Source: CAD feature listing. Evaluate the final solid. Frame: model axes, mm. Give positions to 0.01 mm unless a question says otherwise; leave off trailing zeros. Write each loop counter-clockwise with the first axis right and the second up, starting at its lowest first coordinate (ties: lowest second). Pieces come first, ordered by that corner, then holes. Notation, with made-up numbers: (32, -16.5) -> (40, -16.5) arc R21 ccw to (40, 3.5) -> close; hole circle Ø5 at (38, 31). An arc over 180 degrees is marked (long way). Answer as a JSON object with one key per item and string values. Group by question number.
Item 1: Section query B-B on x = 527. Return the cut outline in (y, z).
Item 2: First-contact query: pin 1 Ø4 at (x, z) = (226, -261.85) entering from -Y. Flat tip, straight axial feed; report the tip coordinate or a pass-through.
Item 3: Section query A-A on z = -142. Return the cut outline in (x, y), plus the area to 3 significant figures.
Item 4: Section query C-C on y = 0.45. Give the number of separate pieces and of enclosed holes in the cut face, plus the area to 3 significant figures.
Item 5: Ray query, probe 1 along X at (y, z) = (1.55, -261.85) (3 decimals); probe 2 along Z at (x, y) = (603.8, 1.6) (3 decimals); probe 3 along Z at (x, y) = (133.5, 1.85). Return the intervals inside material, ascending. Write a range as from..to.
from build123d import *

# Parameters (mm, degrees)
EXTRUDE_1_DEPTH     = 2
SKETCH_2_R          = 1.525
SKETCH_2_R_2        = 1.75
CUT_EXTRUDE_1_DEPTH = 2
SKETCH_3_W          = 2
SKETCH_3_H          = 6
CUT_EXTRUDE_2_DEPTH = 10
FILLET_2_R          = 1


with BuildPart() as part:
    # 草图1 → 凸台-拉伸1 (new body)
    with BuildSketch(Plane(origin=(0, 0, 0), x_dir=(1, 0, 0), z_dir=(0, 1, 0))):
        Polygon((0, 0), (0, 372.1), (608.8, 372.1), (608.8, 17), (125.65, 17), (117.15, 0), align=None)
    extrude(amount=EXTRUDE_1_DEPTH)

    # 草图2 → 切除-拉伸1 (cut)
    with BuildSketch(Plane(origin=(0, 2, 0), x_dir=(1, 0, 0), z_dir=(0, 1, 0))):
        with Locations(Location((5, 349.1, 0), (0, 0, 270))):
            Circle(SKETCH_2_R)
        with Locations(Location((26, 366.1, 0), (0, 0, 270))):
            Circle(SKETCH_2_R)
        with Locations(Location((129.25, 366.1, 0), (0, 0, 270))):
            Circle(SKETCH_2_R)
        with Locations(Location((5, 223.05, 0), (0, 0, 270))):
            Circle(SKETCH_2_R)
        with Locations(Location((603.8, 223.05, 0), (0, 0, 90))):
            Circle(SKETCH_2_R)
        with Locations(Location((479.55, 366.1, 0), (0, 0, 90))):
            Circle(SKETCH_2_R)
        with Locations(Location((582.8, 366.1, 0), (0, 0, 90))):
            Circle(SKETCH_2_R)
        with Locations(Location((603.8, 349.1, 0), (0, 0, 90))):
            Circle(SKETCH_2_R)
        with Locations(Location((10.2, 71.95, 0), (0, 0, 270))):
            Circle(SKETCH_2_R)
        with Locations(Location((598.6, 71.95, 0), (0, 0, 90))):
            Circle(SKETCH_2_R)
        with Locations(Location((9.2, 6, 0), (0, 0, 270))):
            Circle(SKETCH_2_R_2)
        with Locations(Location((102.4, 6, 0), (0, 0, 270))):
            Circle(SKETCH_2_R_2)
        with Locations(Location((62, 261.85, 0), (0, 0, 270))):
            Circle(SKETCH_2_R)
        with Locations(Location((62, 127.85, 0), (0, 0, 270))):
            Circle(SKETCH_2_R)
        with Locations(Location((226, 261.85, 0), (0, 0, 270))):
            Circle(SKETCH_2_R)
        with Locations(Location((226, 127.85, 0), (0, 0, 270))):
            Circle(SKETCH_2_R)
        Polygon((70, 271.85), (75, 271.85), (94, 271.85), (155, 271.85), (184, 271.85), (218, 271.85), (218, 117.85), (70, 117.85), align=None)
    extrude(amount=-CUT_EXTRUDE_1_DEPTH, mode=Mode.SUBTRACT)

    # 草图3 → 切除-拉伸2 (cut)
    with BuildSketch(Plane(origin=(0, 2, 0), x_dir=(1, 0, 0), z_dir=(0, 1, 0))):
        with Locations((65, 250.330488495)):
            Rectangle(SKETCH_3_W, SKETCH_3_H)
        with Locations((60.132371309, 250.330488495)):
            Rectangle(SKETCH_3_W, SKETCH_3_H)
        with Locations((227.867628691, 250.647738708)):
            Rectangle(SKETCH_3_W, SKETCH_3_H)
        with Locations((223, 250.647738708)):
            Rectangle(SKETCH_3_W, SKETCH_3_H)
    extrude(amount=-CUT_EXTRUDE_2_DEPTH, mode=Mode.SUBTRACT)

    # 圆角2
    fillet_2_edges = [part.edges().sort_by_distance(p)[0] for p in [
        (61.132371309, 1, -247.330488495),
        (59.132371309, 1, -247.330488495),
        (66, 1, -247.330488495),
        (64, 1, -247.330488495),
        (59.132371309, 1, -253.330488495),
        (61.132371309, 1, -253.330488495),
        (228.867628691, 1, -247.647738708),
        (222, 1, -247.647738708),
        (228.867628691, 1, -253.647738708),
        (224, 1, -253.647738708),
        (226.867628691, 1, -253.647738708),
        (222, 1, -253.647738708),
        (64, 1, -253.330488495),
        (66, 1, -253.330488495),
        (224, 1, -247.647738708),
        (226.867628691, 1, -247.647738708),
    ]]
    fillet(fillet_2_edges, radius=FILLET_2_R - 0.0001)  # a hair under: the kernel refuses the full size


solid = part.part
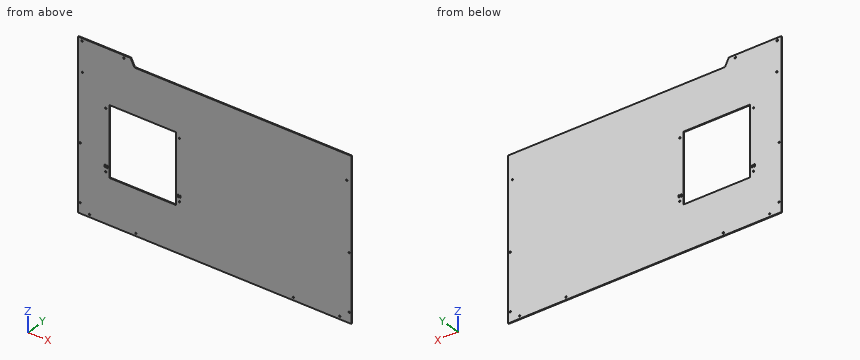
Worked answers:
{
 "1": {"outline": "(0, -372.1) -> (2, -372.1) -> (2, -17) -> (0, -17) -> close"},
 "2": {"pin 1": "y = 0"},
 "3": {"outline": "(0, 0) -> (70, 0) -> (70, 2) -> (0, 2) -> close; (218, 0) -> (608.8, 0) -> (608.8, 2) -> (218, 2) -> close", "area": "922 mm^2"},
 "4": {"separate pieces": "1", "enclosed holes": "21", "area": "195,000 mm^2"},
 "5": {"probe 1": "0..60.475, 63.525..70, 218..224.475, 227.525..608.8", "probe 2": "-372.1..-350.625, -347.575..-224.575, -221.525..-17", "probe 3": "-372.1..-271.85, -117.85..-17"}
}
